```python
from build123d import *

# Parameters (mm, degrees)
F0_W     = 96
F0_H     = 80
F1_DEPTH = 80
F2_W     = 94
F2_H     = 78
F2_W_2   = 60
F2_H_2   = 50
F3_DEPTH = 10
F4_R     = 9.99999


# Not quite as in the source:
# - a fillet or chamfer is up to 0.001 mm smaller than in the source, because OpenCascade refuses the exact size
# - a pattern or mirror of a feature is missing from the dataset's text; its kind, count and spacing are read off the source's solid


with BuildPart() as f1:
    # F0 (on Top) → F1 (new body)
    with BuildSketch(Plane.XY):
        Rectangle(F0_W, F0_H)
    extrude(amount=F1_DEPTH)

    # F2 (on face) → F3 (cut)
    with BuildSketch(Plane.XZ.offset(40)):
        with Locations((0, 40)):
            Rectangle(F2_W, F2_H)
        with Locations((0, 40)):
            Rectangle(F2_W_2, F2_H_2, mode=Mode.SUBTRACT)
    f3 = extrude(amount=-F3_DEPTH, mode=Mode.SUBTRACT)

    # F3_copies: F3 across plane
    add(f3.mirror(Plane.ZX), mode=Mode.SUBTRACT)

    # F4 (radius 10 in the source; OpenCascade refuses exactly that, so slightly less here)
    f4_edges = [f1.edges().sort_by_distance(p)[0] for p in [
        (30, -40, 40),
        (-30, -40, 40),
        (30, 40, 40),
        (-30, 40, 40),
    ]]
    fillet(f4_edges, radius=F4_R)


solid = f1.part
```
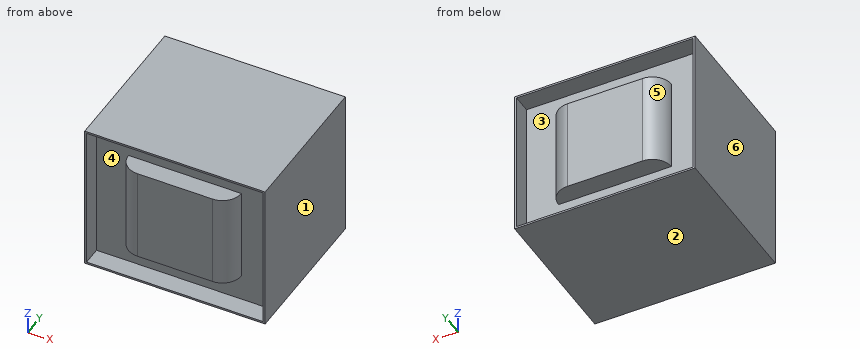
The model under review builds one solid part; all positions refer to its coordinate system, in mm. Face numbers are marked on the shaded views. A direction names the side the tool comes from. Round coordinates to 2 decimals unless told otherwise and drop trailing zeros. Write each loop counter-clockwise with the first axis right and the second up, starting at its lowest first coordinate (ties: lowest second). Pieces come first, ordered by that corner, then holes.
(1) Machinability: for the marked faces 4, 5 and 6, which of the approach directions +Z, -Z, +X, -X, +Y, -Y give a long, thin tool a straight path to every point of the face, cutting with its end or side? Answer none if there is none.
(2) We need section C-C on y = 31.5. Give the boundary of the cut face in (x, z), and give its area (3 significant figures).
(3) We need section A-A on x = 7.5. Give the boundary of the cut face in (y, z).
(4) Mouldability with a two-part tool opening along Z and no side actions: class the marked faces 1, 2 and 3 as +Z half, -Z half, draft (parallel to the pull), parting line (faces both ways), or undercut.
(5) Wall thickness on L1, parallel to Z at x = 22, y = 37; L2, parallel to X at y = -36, z = 47; L3, parallel to Z at x = 42.5, y = 33.5: over which ranges is each line inside the solid? List them lowest first.
(6) Insertion check: pin 1 (6 mm diameter, centred on x = 33.5, z = 61.5, fed in from +Y). The pin has a flat end and moves straight along its axis. Give the tip position at first contact, or say it passes through.
(7) We need section B-B on z = 7.5. Give the boundary of the cut face in (x, y), and give its area (3 significant figures).
Findings below:
1. face 4: -Y
1. face 5: +Y
1. face 6: +Z, -Z, -X, +Y, -Y
2. outline: (-48, 0) - (48, 0) - (48, 80) - (-48, 80) - close; (-29.89, 15) - (29.89, 15) - (29.89, 65) - (-29.89, 65) - close; hole (-47, 1) - (47, 1) - (47, 79) - (-47, 79) - close
2. area: 3,340 mm2
3. outline: (-40, 0) - (40, 0) - (40, 1) - (30, 1) - (30, 15) - (40, 15) - (40, 65) - (30, 65) - (30, 79) - (40, 79) - (40, 80) - (-40, 80) - (-40, 79) - (-30, 79) - (-30, 65) - (-40, 65) - (-40, 15) - (-30, 15) - (-30, 1) - (-40, 1) - close
4. face 1: draft
4. face 2: -Z half
4. face 3: undercut
5. L1: z = 0 to 1, 15 to 65, 79 to 80
5. L2: x = -48 to -47, -28 to 28, 47 to 48
5. L3: z = 0 to 1, 79 to 80
6. pin 1: stops at y = 30
7. outline: (-48, -40) - (-47, -40) - (-47, -30) - (47, -30) - (47, -40) - (48, -40) - (48, 40) - (47, 40) - (47, 30) - (-47, 30) - (-47, 40) - (-48, 40) - close
7. area: 5,800 mm2
